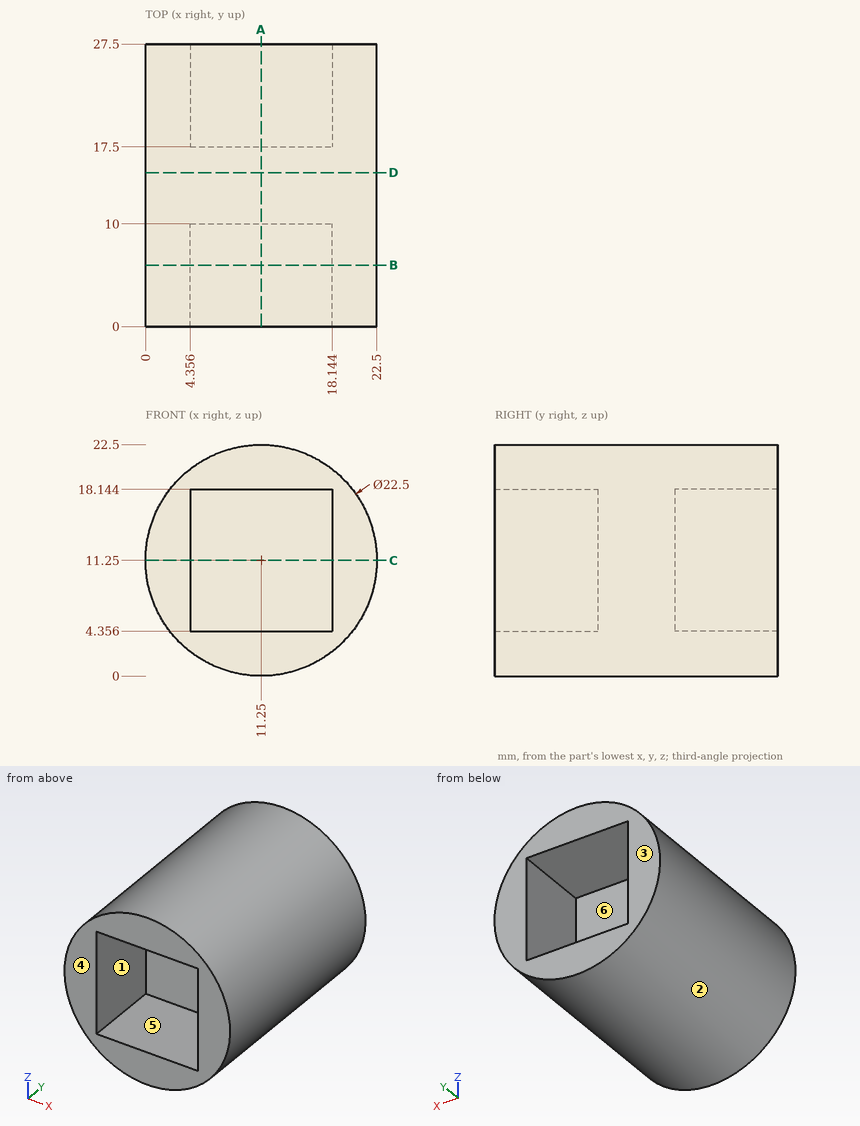
Design review of the part shown in the three views and the two pictorial views. Dimensions are in mm from the part's minimum x, y and z. A direction names the side the tool comes from. Coordinates: 2 decimals unless noted, no trailing zeros. Write each loop counter-clockwise with the first axis right and the second up, starting at its lowest first coordinate (ties: lowest second). Pieces come first, ordered by that corner, then holes.
1) Clearance check with flat-ended pins moving along their axes: pin 1 Ø3 at (x, y) = (17.5, 5.5) entering from +Z; pin 2 Ø4 at (x, y) = (18.5, 5.5) entering from -Z; pin 3 Ø1.5 at (x, y) = (18, 24.5) entering from -Z. State where each tip first meets the part, or that it passes through.
2) We need section B-B on y = 6. State the section outline as (x, z) points.
3) We need section C-C on z = 11.25. State the section outline as (x, y) points, then the cut area to 3 significant figures.
4) We need section D-D on y = 15. State the section outline as (x, z) points, then the cut area to 3 significant figures.
5) We need section A-A on x = 11.25. State the section outline as (y, z) points, then the cut area to 3 significant figures.
6) The part is to be moulded in two halves that separate along X. For the marked faces 1, 2 and 3, say which applies: pulls with the +X half, pulls with the -X half, needs draft (parallel to the pull), parting line crosses it, or undercut.
7) To check wall thickness, follow probe 1 along Z at (x, y) = (11.5, 20); probe 2 along Y at (x, z) = (13.5, 6.75); probe 3 along Z at (x, y) = (7, 6.75) (1 decimal). State the ranges of each line that lie inside material, in increasing order.
8) Machinability: for the marked faces 4, 5 and 6, which of the approach directions +Z, -Z, +X, -X, +Y, -Y give a long, thin tool a straight path to every point of the face, cutting with its end or side? Answer none if there is none.
Answer list:
1. pin 1: stops at z = 21.45
1. pin 2: stops at z = 1.3
1. pin 3: stops at z = 1.73
2. outline: circle Ø22.5 at (11.25, 11.25); hole (4.36, 4.36) - (18.14, 4.36) - (18.14, 18.14) - (4.36, 18.14) - close
3. outline: (0, 0) - (4.36, 0) - (4.36, 10) - (18.14, 10) - (18.14, 0) - (22.5, 0) - (22.5, 27.5) - (18.14, 27.5) - (18.14, 17.5) - (4.36, 17.5) - (4.36, 27.5) - (0, 27.5) - close
3. area: 343 mm2
4. outline: circle Ø22.5 at (11.25, 11.25)
4. area: 398 mm2
5. outline: (0, 0) - (27.5, 0) - (27.5, 4.36) - (17.5, 4.36) - (17.5, 18.14) - (27.5, 18.14) - (27.5, 22.5) - (0, 22.5) - (0, 18.14) - (10, 18.14) - (10, 4.36) - (0, 4.36) - close
5. area: 343 mm2
6. face 1: undercut
6. face 2: parting line crosses it
6. face 3: needs draft
7. probe 1: z = 0 to 4.36, 18.14 to 22.5
7. probe 2: y = 10 to 17.5
7. probe 3: z = 0.8 to 4.4, 18.1 to 21.7
8. face 4: +Z, -Z, +X, -X, -Y
8. face 5: -Y
8. face 6: +Y
